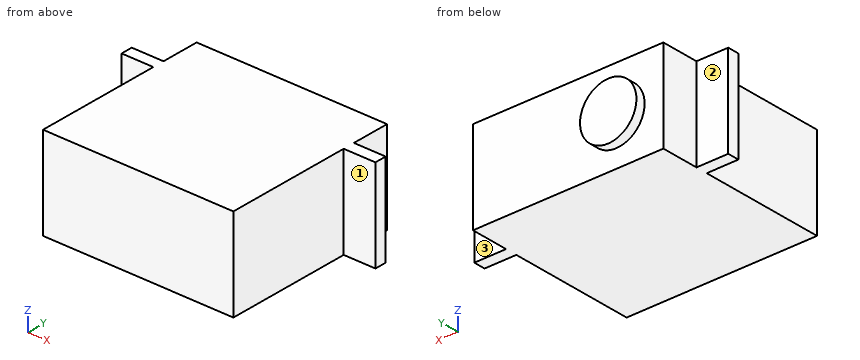
from build123d import *

# Parameters (mm, degrees)
SKETCH1_W           = 40.5
SKETCH1_H           = 19.6
BOSS_EXTRUDE1_DEPTH = 37.6
SKETCH2_R           = 6
BOSS_EXTRUDE2_DEPTH = 2
SKETCH3_W           = 6.75
SKETCH3_H           = 2.5
BOSS_EXTRUDE3_DEPTH = 19.6


with BuildPart() as part:
    # Sketch1 → Boss-Extrude1 (new body)
    with BuildSketch(Plane(origin=(0, 0, 0), x_dir=(1, 0, 0), z_dir=(0, 1, 0))):
        Rectangle(SKETCH1_W, SKETCH1_H)
    extrude(amount=BOSS_EXTRUDE1_DEPTH)

    # Sketch2 → Boss-Extrude2 (add)
    with BuildSketch(Plane(origin=(0, 37.6, 0), x_dir=(1, 0, 0), z_dir=(0, 1, 0))):
        with Locations(Location((-10.25, 0, 0), (0, 0, 90))):
            Circle(SKETCH2_R)
    extrude(amount=BOSS_EXTRUDE2_DEPTH)

    # Sketch3 → Boss-Extrude3 (add)
    with BuildSketch(Plane.XY.offset(9.8)):
        with Locations((-23.625, 28.25)):
            Rectangle(SKETCH3_W, SKETCH3_H)
        with Locations((23.625, 28.25)):
            Rectangle(SKETCH3_W, SKETCH3_H)
    extrude(amount=-BOSS_EXTRUDE3_DEPTH)


solid = part.part
Design review of the part built by this model. Coordinates are the model's own, in mm. Face numbers are marked on the shaded views. A direction names the side the tool comes from. Coordinates: 2 decimals unless noted, no trailing zeros. Order: outer loops, then holes, each group sorted by start corner. A loop starts at its lowest first (then second) coordinate and runs counter-clockwise, first axis right, second up. Notation, with made-up numbers: (65.25, 21.25) - (119.25, 21.25) arc R15 ccw to (119.25, 39.25) - close; hole circle Ø1 at (-8, 23). An arc over 180 degrees is marked (long way). Put each result on its own line as item: value.
1) Take a section at C-C, the plane y = 24. Give the boundary of the cut face in (x, z), and give its area (3 significant figures).
Response values:
outline: (-20.25, -9.8) - (20.25, -9.8) - (20.25, 9.8) - (-20.25, 9.8) - close
area: 794 mm²
2) Take a section at B-B, the plane z = 0. Give the boundary of the cut face in (x, y), and give its area (3 significant figures).
Response values:
outline: (-27, 27) - (-20.25, 27) - (-20.25, 0) - (20.25, 0) - (20.25, 27) - (27, 27) - (27, 29.5) - (20.25, 29.5) - (20.25, 37.6) - (-4.25, 37.6) - (-4.25, 39.6) - (-16.25, 39.6) - (-16.25, 37.6) - (-20.25, 37.6) - (-20.25, 29.5) - (-27, 29.5) - close
area: 1,580 mm²
3) Take a section at D-D, the plane z = -7.25. Give the boundary of the cut face in (x, y), and give its area (3 significant figures).
Response values:
outline: (-27, 27) - (-20.25, 27) - (-20.25, 0) - (20.25, 0) - (20.25, 27) - (27, 27) - (27, 29.5) - (20.25, 29.5) - (20.25, 37.6) - (-20.25, 37.6) - (-20.25, 29.5) - (-27, 29.5) - close
area: 1,560 mm²
4) Take a section at A-A, the plane x = -10.25. Give the boundary of the cut face in (y, z), and give its area (3 significant figures).
Response values:
outline: (0, -9.8) - (37.6, -9.8) - (37.6, -6) - (39.6, -6) - (39.6, 6) - (37.6, 6) - (37.6, 9.8) - (0, 9.8) - close
area: 761 mm²
5) Insertion check: P1, Ø5.5, axis at x = 23.5, z = -0.5, coming from the +Y side; P2, Ø10, axis at y = 35, z = -5.5, coming from the +X side; P3, Ø5, axis at y = 8.5, z = 6.5, coming from the -X side. Each pin has a flat end and moves straight along its axis. Give the tip position at first contact, or say it passes through.
Response values:
P1: stops at y = 29.5
P2: stops at x = 20.25
P3: stops at x = -20.25
6) Tool access review of the marked faces 1, 2 and 3: name each direction out of +Z, -Z, +X, -X, +Y, -Y from which nothing blocks a thin tool from reaching the whole face with its end or side.
Response values:
face 1: +Z, -Z, +X, -Y
face 2: +Z, -Z, -X, +Y
face 3: +Z, -Z, +X, +Y
7) Wall thickness on L1, parallel to Y at x = -3, z = -8.25; L2, parallel to Y at x = 24.5, z = -1.75; L3, parallel to X at y = 37, z = 4.25: over which ranges is each line inside the solid? List them lowest first. Write a range as from..to.
Response values:
L1: y = 0..37.6
L2: y = 27..29.5
L3: x = -20.25..20.25
